```python
from build123d import *

# Parameters (mm, degrees)
F0_R     = 10
F1_DEPTH = 13.925
F2_R     = 7.5
F3_DEPTH = 6


with BuildPart() as f1:
    # F0 (on Top) → F1 (new body, symmetric)
    with BuildSketch(Plane.XY):
        with Locations((-54.4874072075, -46.7285439372)):
            Circle(F0_R)
    extrude(amount=F1_DEPTH, both=True)

    # F2 (on face) → F3 (join)
    with BuildSketch(Plane.XY.offset(13.925)):
        with Locations((-54.4874072075, -46.7285439372)):
            Circle(F2_R)
    extrude(amount=F3_DEPTH)

    # F4: F1 across plane


with BuildPart() as f1_1:
    add(f1.part)
    add(f1.part.mirror(Plane.XY))


solid = f1_1.part
```
Verification items for the finished model (mm, model axes). A direction names the side the tool comes from. Coordinates: 2 decimals unless noted, no trailing zeros. Loops run counter-clockwise (first coordinate to the right, second up) from the corner with the lowest first, then second, coordinate; pieces in that order, holes last. Notation, with made-up numbers: (1.5, 83) - (8.5, 83) arc R9 ccw to (8.5, 91) - close; hole circle Ø2 at (11.25, -12). An arc over 180 degrees is marked (long way). Put each result on its own line as item: value.
Item 1: Section check D-D (z = -16). Enter the section's corners in (x, y), then the cut area to 3 significant figures.
Conclusion:
outline: circle Ø15 at (-54.49, -46.73)
area: 177 mm2
Item 2: Set-up check for faces 1 (the face through (-55, -47, 19.925)), 2 (the face through (-61.98, -46.4, -16.88)), 3 (the face through (-53, -39, 13.925)): record each of +Z, -Z, +X, -X, +Y, -Y from which the full face is reachable in a straight line by a thin tool's end or side.
Conclusion:
face 1: +Z, +X, -X, +Y, -Y
face 2: -Z
face 3: +Z
Item 3: Section check B-B (x = -57.75). Enter the section's corners in (y, z) (3 decimals), then the cut area to 3 significant figures.
Conclusion:
outline: (-56.181, -13.925) - (-53.482, -13.925) - (-53.482, -19.925) - (-39.975, -19.925) - (-39.975, -13.925) - (-37.276, -13.925) - (-37.276, 13.925) - (-39.975, 13.925) - (-39.975, 19.925) - (-53.482, 19.925) - (-53.482, 13.925) - (-56.181, 13.925) - close
area: 689 mm2
Item 4: Scan lines: line 1 along Z through (x, y) = (-46.5, -41.25) (3 decimals); line 2 along X through (y, z) = (-46.25, -11); line 3 along Y through (x, z) = (-47.5, -13.5). Record each from-to range of solid material in increasing order.
Conclusion:
line 1: z = -13.925 to 13.925
line 2: x = -64.48 to -44.5
line 3: y = -53.88 to -39.57
Item 5: Section check C-C (z = -4). Enter the section's corners in (x, y), then the cut area to 3 significant figures.
Conclusion:
outline: circle Ø20 at (-54.49, -46.73)
area: 314 mm2
Item 6: Gauge pin test, flat ends, axial feed: pin 1 Ø10 at (y, z) = (-53, -13.5) entering from -X; pin 2 Ø6 at (y, z) = (-40, -10.5) entering from -X; pin 3 Ø5 at (y, z) = (-42, -1) entering from +X. Record the tip position at first contact, or that the pin passes through.
Conclusion:
pin 1: stops at x = -64.41
pin 2: stops at x = -63.77
pin 3: stops at x = -44.74
Item 7: Section check A-A (y = -39.75). Enter the section's corners in (x, z) (3 decimals), then the cut area to 3 significant figures.
Conclusion:
outline: (-61.65, -13.925) - (-57.235, -13.925) - (-57.235, -19.925) - (-51.74, -19.925) - (-51.74, -13.925) - (-47.325, -13.925) - (-47.325, 13.925) - (-51.74, 13.925) - (-51.74, 19.925) - (-57.235, 19.925) - (-57.235, 13.925) - (-61.65, 13.925) - close
area: 465 mm2
